Autodesk Inventor part; units mm, degrees
ref_plane "YZ Plane" through (0, 0, 0) normal (1, 0, 0) x (0, 1, 0)
ref_plane "XZ Plane" through (0, 0, 0) normal (0, 1, 0) x (-1, 0, 0)
ref_plane "XY Plane" through (0, 0, 0) normal (0, 0, 1) x (1, 0, 0)
sketch "Sketch1" plane through (0, 0, 0) normal (1, 0, 0) x (0, 1, 0)
  line L0 (0, 0) -> (-25.4, 0)
  line L1 (-25.4, 0) -> (-25.4, -101.6)
  line L2 (-25.4, -101.6) -> (0, -101.6)
  line L3 (0, -101.6) -> (0, 0)
  line L4 (-3.175, -3.175) -> (-22.225, -3.175)
  line L5 (-22.225, -3.175) -> (-22.225, -98.425)
  line L6 (-22.225, -98.425) -> (-3.175, -98.425)
  line L7 (-3.175, -98.425) -> (-3.175, -3.175)
  dimension "d0" = 25.4
  dimension "d1" = 101.6
  dimension "d2" = 3.175
extrude "Extrusion1" add sketch "Sketch1" along normal blind 127
sketch "Sketch2" plane through (0, 0, 0) normal (0, 1, 0) x (1, 0, 0)
  circle A0 centre (63.5, 50.8) radius 41
  point P0 (0, 0)
extrude "Extrusion2" cut sketch "Sketch2" against normal blind 127
sketch "Sketch3" plane through (0, 0, 0) normal (0, 1, 0) x (1, 0, 0)
  circle A0 centre (63.5, 50.8) radius 49.5
  circle A1 centre (31.251, 82.8975) radius 2.55
  circle A2 centre (63.3929, 96.2999) radius 2.55
  circle A3 centre (95.5975, 83.049) radius 2.55
  circle A4 centre (108.9999, 50.9071) radius 2.55
  circle A5 centre (95.749, 18.7025) radius 2.55
  circle A6 centre (63.6071, 5.3001) radius 2.55
  circle A7 centre (31.4025, 18.551) radius 2.55
  circle A8 centre (18.0001, 50.6929) radius 2.55
  circle A9 centre (63.5, 50.8) radius 29
  point P0 (0, 0)
extrude "Extrusion3" cut sketch "Sketch3" against normal blind 127 contours A1 | A2 | A3 | A4 | A5 | A6 | A7 | A8
sketch "Sketch4" plane through (0, 0, 0) normal (0, 1, 0) x (1, 0, 0)
  circle A0 centre (31.4025, 18.551) radius 2.55
  circle A1 centre (95.749, 18.7025) radius 2.55
  circle A2 centre (95.5975, 83.049) radius 2.55
  circle A3 centre (31.251, 82.8975) radius 2.55
  circle A4 centre (63.3929, 96.2999) radius 2.55
  circle A5 centre (108.9999, 50.9071) radius 2.55
  circle A6 centre (63.6071, 5.3001) radius 2.55
  circle A7 centre (18.0001, 50.6929) radius 2.55
  circle A8 centre (63.5, 50.8) radius 41
  line L0 (0, 101.6) -> (0, 0)
  line L1 (0, 0) -> (127, 0)
  line L2 (127, 101.6) -> (127, 0)
  line L3 (0, 101.6) -> (127, 101.6)
  line L4 (0, 101.6) -> (127, 101.6)
  line L5 (127, 0) -> (113.4618, 0)
  line L6 (113.4618, 0) -> (113.4618, 101.6)
  line L7 (113.4618, 101.6) -> (127, 101.6)
  line L8 (127, 101.6) -> (127, 0)
  dimension "d9" = 13.5382
extrude "Extrusion4" cut sketch "Sketch4" against normal blind 127 contours L3 L2 L1 L6
sketch "Sketch6" plane through (0, 0, 0) normal (0, 1, 0) x (1, 0, 0)
  circle A0 centre (10.2546, 88.1171) radius 3.175
  circle A1 centre (-15.1454, 88.2911) radius 3.175
  arc A2 (59.2572, 91.5755) -> (37.6675, 82.6327) centre (63.5, 50.8) ccw
  arc A3 (58.9842, 100.7643) -> (59.2572, 91.5755) centre (63.5, 96.3) ccw
  line L0 (-60.4471, 100.7643) -> (58.9842, 100.7643)
  line L1 (-60.4471, 100.7643) -> (-35.0471, 75.3643)
  line L2 (-35.0471, 75.3643) -> (30.6788, 75.3643)
  arc A4 (31.6673, 76.6325) -> (30.6788, 75.3643) centre (63.5, 50.8) ccw
  arc A5 (37.6675, 82.6327) -> (31.6673, 76.6325) centre (31.3266, 82.9734) ccw
  circle A6 centre (63.5, 50.8) radius 9.525
  circle A7 centre (-15.1454, 88.2911) radius 3.175
  circle A8 centre (100.7643, -2.7658) radius 3.175
  circle A9 centre (10.2546, 88.1171) radius 3.175
  line L3 (113.4643, 100.7643) -> (113.4643, -13.5357)
  line L4 (-35.8911, 100.7643) -> (113.4643, 100.7643)
  line L5 (-35.8911, 100.7643) -> (-4.2078, -13.5357)
  line L6 (113.4643, -13.5357) -> (-4.2078, -13.5357)
  line L7 (91.2393, -13.5357) -> (91.2393, 100.7643)
  line L8 (110.2893, -13.5357) -> (91.2393, -13.5357)
  line L9 (110.2893, -13.5357) -> (110.2893, 100.7643)
  line L10 (91.2393, 100.7643) -> (110.2893, 100.7643)
  line L11 (113.4618, 0) -> (113.4618, 101.6)
  line L12 (0, 101.6) -> (113.4618, 101.6)
  line L13 (0, 101.6) -> (0, 0)
  line L14 (0, 0) -> (113.4618, 0)
  circle A10 centre (63.5, 50.8) radius 41
  circle A11 centre (18.0001, 50.6929) radius 2.55
  circle A12 centre (63.6071, 5.3001) radius 2.55
  circle A13 centre (108.9999, 50.9071) radius 2.55
  circle A14 centre (63.3929, 96.2999) radius 2.55
  circle A15 centre (31.251, 82.8975) radius 2.55
  circle A16 centre (95.5975, 83.049) radius 2.55
  circle A17 centre (95.749, 18.7025) radius 2.55
  circle A18 centre (31.4025, 18.551) radius 2.55
  circle A19 centre (100.7643, 9.8) radius 3.175
  circle A20 centre (10.2546, 9.8) radius 3.175
  circle A21 centre (100.7643, 91.8) radius 3.175
  circle A22 centre (10.2546, 9.8) radius 3.175
  circle A23 centre (100.7643, 9.8) radius 3.175
  circle A24 centre (100.7643, 91.8) radius 3.175
  dimension "d12" = 6.35
  dimension "d13" = 6.35
  dimension "d14" = 6.35
extrude "Extrusion5" cut sketch "Sketch6" against normal blind 127 contours A0 | A19 | A20 | A21
properties part number "4x1x5 box beam"
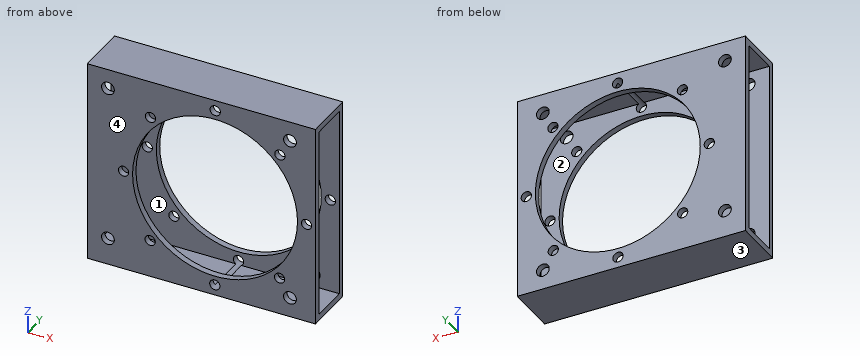
The listing builds one solid part. Answer for the finished solid, in the listing's coordinates (mm). Face numbers are marked on the shaded views. Give positions to 0.01 mm unless a question says otherwise; leave off trailing zeros. Order: outer loops, then holes, each group sorted by start corner. A loop starts at its lowest first (then second) coordinate and runs counter-clockwise, first axis right, second up. Notation, with made-up numbers: M 46,13 L 53,13 A19 ccw 53,22 Z; hole C 44.5,-1.5 d11. An arc over 180 degrees is marked long. Put each result on its own line as item: value. Start each with the question number.
Item 1: The part is cut by section B-B, the plane x = 59.5. Determine the outline of the cut face in (y, z) (3 decimals), and give its area (3 significant figures).
Item 2: The part is cut by section C-C, the plane z = -11.5. State how many separate pieces and enclosed holes the cut face has, and give its area (3 significant figures).
Item 3: The part is cut by section D-D, the plane z = -72.5. Determine the outline of the cut face in (x, y) (3 decimals), and give its area (3 significant figures).
Item 4: Find the intervals of material crossed by line 1 along Z through (x, y) = (63.5, -0.8); line 2 along Z through (x, y) = (40, -5.25) (3 decimals); line 3 along Y through (x, z) = (36, -15) (3 decimals), in increasing order.
Item 5: The part is cut by section A-A, the plane y = -9.25. Determine the outline of the cut face in (x, z) (3 decimals).
Item 6: Flat-ended cylindrical pins translate along their axes: P1, Ø12, axis at x = 24, z = -75.5, coming from the +Y side; P2, Ø4.5, axis at x = 95.6, z = -83.05, coming from the +Y side. Find the tip coordinate at first contact, or state that the pin passes through.
Item 7: For a pull along Z with two mould halves and no side action, classify the marked faces 1, 2, 3 and 4 as +Z half, -Z half, draft (parallel to the pull), parting line (faces both ways), or undercut.
Answer key:
1. outline: M -25.4,-101.6 L 0,-101.6 L 0,-91.604 L -3.175,-91.604 L -3.175,-98.425 L -22.225,-98.425 L -22.225,-91.604 L -25.4,-91.604 Z; M -25.4,-9.996 L -22.225,-9.996 L -22.225,-3.175 L -3.175,-3.175 L -3.175,-9.996 L 0,-9.996 L 0,0 L -25.4,0 Z
1. area: 248 mm²
2. separate pieces: 8
2. enclosed holes: 0
2. area: 504 mm²
3. outline: M 0,-25.4 L 28.713,-25.4 L 28.713,-22.225 L 0,-22.225 Z; M 0,-3.175 L 28.713,-3.175 L 28.713,0 L 0,0 Z; M 98.287,-25.4 L 113.462,-25.4 L 113.462,-22.225 L 98.287,-22.225 Z; M 98.287,-3.175 L 113.462,-3.175 L 113.462,0 L 98.287,0 Z
3. area: 279 mm²
4. line 1: z = -101.6 to -98.85, -93.75 to -91.8, -9.8 to -7.85, -2.75 to 0
4. line 2: z = -101.6 to -98.425, -3.175 to 0
4. line 3: y = -25.4 to -22.225, -3.175 to 0
5. outline: M 0,-101.6 L 113.462,-101.6 L 113.462,-98.425 L 64.802,-98.425 A2.55 cw 61.983,-98.425 L 0,-98.425 Z; M 0,-3.175 L 62.198,-3.175 A2.55 cw 65.017,-3.175 L 113.462,-3.175 L 113.462,0 L 0,0 Z
6. P1: stops at y = 0
6. P2: passes through
7. face 1: undercut
7. face 2: undercut
7. face 3: -Z half
7. face 4: draft
